Check sheet for the modelled part. Datum: model origin and axes. Units: mm. A direction names the side the tool comes from. Round coordinates to 2 decimals unless told otherwise and drop trailing zeros. Write each loop counter-clockwise with the first axis right and the second up, starting at its lowest first coordinate (ties: lowest second). Pieces come first, ordered by that corner, then holes.
Item 1: Set-up check for faces 3 (the flat face through (0, 0.5, -1.2)), 4 (the flat face through (0.5, 0, 1.3)), 5 (the cylindrical face through (9.484, 1.972, 0.545)): record each of +Z, -Z, +X, -X, +Y, -Y from which the full face is reachable in a straight line by a thin tool's end or side.
Item 2: Section check C-C, the plane x = 15. Record the cut outline in (y, z).
Item 3: Section check D-D, the plane z = -19. Record the cut outline in (x, y).
Item 4: Material ranges on line 1 along X through (y, z) = (2.5, 0); line 2 along X through (y, z) = (0.25, 0); line 3 along X through (y, z) = (4.25, 0), recorded low to high.
Item 5: Section check A-A, the plane z = 0. Record the cut outline in (x, y).
Item 6: Section check B-B, the plane y = 2. Record the cut outline in (x, z) (3 decimals), plus the area to 3 significant figures.
Item 7: Release check for a two-part mould opening along X. For faces 1 (the flat face through (-20, 5.9, 13)), 2 (the flat face through (15, 1.97, -6.47)) record: pulls with the +X half, pulls with the -X half, needs draft (parallel to the pull), parting line crosses it, or undercut.
Item 8: Depth check by flat-ended pin: pin 1 (3 mm diameter, centred on y = 1.5, z = -19.5, fed in from +X); pin 2 (3 mm diameter, centred on y = 5, z = 9, fed in from +X); pin 3 (2 mm diameter, centred on x = -9.5, y = 4.5, fed in from -Z); pin 4 (5 mm diameter, centred on x = 3, z = -15, fed in from +Y). Enter the tip coordinate at first touch or a pass-through.
from build123d import *

# Parameters (mm, degrees)
SKETCH1_R                = 9.5
SKETCH1_R_2              = 3.25
BOSS_EXTRUDE1_DEPTH      = 4
SKETCH1_4_R              = 3.25
SKETCH1_4_R_2            = 2.6
BOSS_EXTRUDE2_DEPTH      = 4.5
SKETCH1_5_W              = 3.934463114
SKETCH1_5_H              = 3.4
SKETCH1_5_R              = 1
BOSS_EXTRUDE3_DEPTH      = 0.5
SKETCH1_6_R              = 30
SKETCH1_6_R_2            = 23.5
BOSS_EXTRUDE4_DEPTH      = 5.9
BOSS_EXTRUDE4_DEPTH_BACK = 1.9


with BuildPart() as part:
    # Sketch1 → Boss-Extrude1 (new body)
    with BuildSketch(Plane(origin=(0, 0, 0), x_dir=(1, 0, 0), z_dir=(0, 1, 0))):
        with BuildLine():
            ThreePointArc((-9.183595688, -2.431372091), (-9.486673449, 0.503017773), (-8.874983612, 3.388903346))
            Line((-8.874983612, 3.388903346), (-23.194055647, 3.779653774))
            ThreePointArc((-23.194055647, 3.779653774), (-23.46703432, 1.244307122), (-23.463699022, -1.305690697))
            Line((-23.463699022, -1.305690697), (-9.183595688, -2.431372091))
        make_face()
        Circle(SKETCH1_R)
        with Locations(Location((0, 0, 0), (0, 0, 270))):
            Circle(SKETCH1_R_2, mode=Mode.SUBTRACT)
        with BuildLine():
            ThreePointArc((-0.525514867, -9.485453818), (-3.409941646, -8.866921561), (-5.965559371, -7.39338227))
            Line((-5.965559371, -7.39338227), (-10.762021714, -20.890880513))
            ThreePointArc((-10.762021714, -20.890880513), (-8.435118809, -21.933963861), (-6.008896103, -22.718784466))
            Line((-6.008896103, -22.718784466), (-0.525514867, -9.485453818))
        make_face()
        with BuildLine():
            Line((19.749996995, -12.735290287), (8.858809639, -3.430960767))
            ThreePointArc((8.858809639, -3.430960767), (7.379213612, -5.983076673), (5.188065158, -7.958264881))
            Line((5.188065158, -7.958264881), (16.54276044, -16.690927986))
            ThreePointArc((16.54276044, -16.690927986), (18.253844197, -14.800242296), (19.749996995, -12.735290287))
        make_face()
        with BuildLine():
            Line((18.215065524, 14.847942212), (6.000560323, 7.365003449))
            ThreePointArc((6.000560323, 7.365003449), (7.970546468, 5.16917682), (9.171959975, 2.474904082))
            Line((9.171959975, 2.474904082), (20.986009934, 10.575319714))
            ThreePointArc((20.986009934, 10.575319714), (19.716614948, 12.78691108), (18.215065524, 14.847942212))
        make_face()
        with BuildLine():
            Line((-6.068306016, 22.702987955), (-2.453144985, 9.177803642))
            ThreePointArc((-2.453144985, 9.177803642), (-0.998421277, 9.44738879), (0.48051785, 9.487839722))
            Line((0.48051785, 9.487839722), (-3.572693012, 23.226835011))
            ThreePointArc((-3.572693012, 23.226835011), (-4.827610123, 22.998786501), (-6.068306016, 22.702987955))
        make_face()
        with BuildLine():
            ThreePointArc((-5.150259407, 7.982783226), (-3.848370829, 8.685622716), (-2.453144985, 9.177803642))
            Line((-2.453144985, 9.177803642), (-6.068306016, 22.702987955))
            ThreePointArc((-6.068306016, 22.702987955), (-7.291125837, 22.340310741), (-8.492467394, 21.911823237))
            Line((-8.492467394, 21.911823237), (-5.150259407, 7.982783226))
        make_face()
    extrude(amount=BOSS_EXTRUDE1_DEPTH)

    # Sketch1_4 → Boss-Extrude2 (add)
    with BuildSketch(Plane(origin=(0, 0, 0), x_dir=(1, 0, 0), z_dir=(0, 1, 0))):
        with Locations(Location((0, 0, 0), (0, 0, 270))):
            Circle(SKETCH1_4_R)
        Circle(SKETCH1_4_R_2, mode=Mode.SUBTRACT)
        with BuildLine():
            ThreePointArc((1.967231557, 1.7), (0, 2.6), (-1.967231557, 1.7))
            Line((-1.967231557, 1.7), (1.967231557, 1.7))
        make_face()
        with BuildLine():
            Line((1.967231557, -1.7), (-1.967231557, -1.7))
            ThreePointArc((-1.967231557, -1.7), (0, -2.6), (1.967231557, -1.7))
        make_face()
    extrude(amount=BOSS_EXTRUDE2_DEPTH)

    # Sketch1_5 → Boss-Extrude3 (add)
    with BuildSketch(Plane(origin=(0, 0, 0), x_dir=(1, 0, 0), z_dir=(0, 1, 0))):
        with BuildLine():
            ThreePointArc((2.6, 0), (2.436678277, 0.906972423), (1.967231557, 1.7))
            Line((1.967231557, 1.7), (1.967231557, -1.7))
            ThreePointArc((1.967231557, -1.7), (2.436678277, -0.906972423), (2.6, 0))
        make_face()
        Rectangle(SKETCH1_5_W, SKETCH1_5_H)
        with Locations(Location((0, 0, 0), (0, 0, 270))):
            Circle(SKETCH1_5_R, mode=Mode.SUBTRACT)
        with BuildLine():
            Line((-1.967231557, -1.7), (-1.967231557, 1.7))
            ThreePointArc((-1.967231557, 1.7), (-2.6, 0), (-1.967231557, -1.7))
        make_face()
    extrude(amount=BOSS_EXTRUDE3_DEPTH)

    # Sketch1_6 → Boss-Extrude4 (add, two sides)
    with BuildSketch(Plane(origin=(0, 0, 0), x_dir=(1, 0, 0), z_dir=(0, 1, 0))) as boss_extrude4_sk:
        with Locations(Location((0, 0, 0), (0, 0, 270))):
            Circle(SKETCH1_6_R)
        with Locations(Location((0, 0, 0), (0, 0, 270))):
            Circle(SKETCH1_6_R_2, mode=Mode.SUBTRACT)
    extrude(amount=BOSS_EXTRUDE4_DEPTH)
    extrude(boss_extrude4_sk.sketch, amount=-BOSS_EXTRUDE4_DEPTH_BACK)


solid = part.part
Values found:
1. face 3: +Y
1. face 4: -Y
1. face 5: +Y, -Y
2. outline: (-1.9, -25.98) - (5.9, -25.98) - (5.9, -18.09) - (-1.9, -18.09) - close; (-1.9, 18.09) - (5.9, 18.09) - (5.9, 25.98) - (-1.9, 25.98) - close; (0, -12.88) - (4, -12.88) - (4, -6.47) - (0, -6.47) - close; (0, 8.68) - (4, 8.68) - (4, 15.5) - (0, 15.5) - close
3. outline: (-23.22, -1.9) - (-13.83, -1.9) - (-13.83, 5.9) - (-23.22, 5.9) - close; (-7.79, 0) - (-2.33, 0) - (-2.33, 4) - (-7.79, 4) - close; (13.83, -1.9) - (23.22, -1.9) - (23.22, 5.9) - (13.83, 5.9) - close
4. line 1: x = -30 to -2.6, 2.6 to 9.5, 23.5 to 30
4. line 2: x = -30 to -1, 1 to 9.5, 23.5 to 30
4. line 3: x = -30 to -23.5, -3.25 to -2.6, 2.6 to 3.25, 23.5 to 30
5. outline: (-30, -1.9) - (-23.5, -1.9) - (-23.5, 0) - (-1, 0) - (-1, 0.5) - (-2.6, 0.5) - (-2.6, 4.5) - (-3.25, 4.5) - (-3.25, 4) - (-23.5, 4) - (-23.5, 5.9) - (-30, 5.9) - close; (1, 0) - (9.5, 0) - (9.5, 4) - (3.25, 4) - (3.25, 4.5) - (2.6, 4.5) - (2.6, 0.5) - (1, 0.5) - close; (23.5, -1.9) - (30, -1.9) - (30, 5.9) - (23.5, 5.9) - close
6. outline: circle Ø60 at (0, 0); hole (-23.464, 1.306) - (-9.184, 2.431) arc R9.5 cw to (-5.966, 7.393) - (-10.762, 20.891) arc R23.5 ccw to start; hole (-23.194, -3.78) arc R23.5 ccw to (-8.492, -21.912) - (-5.15, -7.983) arc R9.5 cw to (-8.875, -3.389) - close; hole (-6.009, 22.719) - (-0.526, 9.485) arc R9.5 cw to (5.188, 7.958) - (16.543, 16.691) arc R23.5 ccw to start; hole (-3.573, -23.227) arc R23.5 ccw to (18.215, -14.848) - (6.001, -7.365) arc R9.5 cw to (0.481, -9.488) - close; hole (-1.967, -1.7) - (1.967, -1.7) arc R2.6 ccw to (1.967, 1.7) - (-1.967, 1.7) arc R2.6 ccw to start; hole (8.859, 3.431) arc R9.5 cw to (9.172, -2.475) - (20.986, -10.575) arc R23.5 ccw to (19.75, 12.735) - close
6. area: 1,740 mm2
7. face 1: needs draft
7. face 2: undercut
8. pin 1: stops at x = 24
8. pin 2: stops at x = 29.05
8. pin 3: stops at z = -28.77
8. pin 4: passes through
